```python
from build123d import *

# Parameters (mm, degrees)
SKETCH_1_W          = 18
SKETCH_1_H          = 49
EXTRUDE_1_DEPTH     = 2
CUT_EXTRUDE_1_DEPTH = 0.1


with BuildPart() as part:
    # ｽｹｯﾁ1 → ﾎﾞｽ - 押し出し1 (new body)
    with BuildSketch(Plane.XY):
        with Locations((9, 24.5)):
            Rectangle(SKETCH_1_W, SKETCH_1_H)
    extrude(amount=EXTRUDE_1_DEPTH)

    # ｽｹｯﾁ2 → ｶｯﾄ - 押し出し1 (cut)
    with BuildSketch(Plane.XY.offset(2)):
        with BuildLine():
            Line((15.875, 36.3125), (15.875, 33.870192308))
            Line((15.875, 33.870192308), (7.775315505, 33.870192308))
            Line((7.775315505, 33.870192308), (6.49214994, 27.607008714))
            add(Edge.make_bspline(
                [(6.49214994, 27.607008714), (6.744262228, 27.676611099), (7.232689912, 27.811454712), (7.953595395, 27.961172542), (8.637981636, 28.051424939), (9.082087281, 28.063748319), (9.29698768, 28.069711538)],
                knots=[0, 0, 0, 0, 1.100273476, 2.13160584, 3.095893838, 4, 4, 4, 4], degree=3))
            add(Edge.make_bspline(
                [(9.29698768, 28.069711538), (9.562896695, 28.063956155), (10.085740255, 28.052639632), (10.850726663, 27.943974013), (11.580973668, 27.772932808), (12.27495408, 27.53398783), (12.933951755, 27.228441252), (13.551903557, 26.846761301), (14.138085072, 26.400900602), (14.68198022, 25.888285431), (15.175404531, 25.324122288), (15.609240996, 24.717530344), (15.977740048, 24.074404643), (16.274108756, 23.388600502), (16.510766458, 22.667699833), (16.668282709, 21.904117441), (16.77317139, 21.105050767), (16.784889768, 20.558692889), (16.790865385, 20.280085637)],
                knots=[0, 0, 0, 0, 1.052922333, 2.070308379, 3.05430497, 4.020497103, 4.973039431, 5.925935799, 6.892292201, 7.88610001, 8.88166317, 9.857072816, 10.836096531, 11.812156883, 12.81219415, 13.836441305, 14.89672472, 16, 16, 16, 16], degree=3))
            add(Edge.make_bspline(
                [(16.790865385, 20.280085637), (16.786340497, 20.086032674), (16.777351873, 19.700549205), (16.731641482, 19.128068125), (16.643632414, 18.567706707), (16.525469862, 18.019390612), (16.372100912, 17.48415792), (16.186437884, 16.960476631), (15.959225626, 16.451606182), (15.710001448, 15.952731619), (15.429378088, 15.475131061), (15.117920743, 15.028483492), (14.788862669, 14.606088649), (14.434795386, 14.212476644), (14.052427901, 13.850233968), (13.646390984, 13.517210839), (13.219924628, 13.20777536), (12.766430926, 12.934488174), (12.296015104, 12.683008062), (11.801883841, 12.47669971), (11.295285147, 12.292251296), (10.76892769, 12.145229331), (10.224003714, 12.030027487), (9.659614974, 11.951782329), (9.078721487, 11.894792638), (8.684964705, 11.891225138), (8.486065204, 11.889423077)],
                knots=[0, 0, 0, 0, 1.056347294, 2.098418968, 3.122841568, 4.141288669, 5.149314143, 6.15115421, 7.162517403, 8.180376062, 9.185164535, 10.17417709, 11.141909838, 12.097768115, 13.052685741, 14.0056014, 14.954263652, 15.917497458, 16.885230207, 17.854509472, 18.828990115, 19.81800267, 20.826176721, 21.857883937, 22.917946725, 24, 24, 24, 24], degree=3))
            add(Edge.make_bspline(
                [(8.486065204, 11.889423077), (8.248796225, 11.894123242), (7.781997537, 11.903370263), (7.098098679, 12.000106743), (6.440093951, 12.138654103), (5.813280227, 12.347090153), (5.212040023, 12.608260854), (4.644467603, 12.938344093), (4.096060448, 13.312398352), (3.589112484, 13.753816468), (3.118603926, 14.236296376), (2.697418571, 14.759883184), (2.322313344, 15.315935282), (1.999295101, 15.90715308), (1.72376392, 16.531983085), (1.507308375, 17.192766359), (1.332603853, 17.886050314), (1.258693796, 18.363344733), (1.221153846, 18.605769231)],
                knots=[0, 0, 0, 0, 1.0467383, 2.05933395, 3.04377827, 4.011590433, 4.970194871, 5.932262533, 6.905835911, 7.896367577, 8.894135286, 9.877477877, 10.858688626, 11.851381753, 12.8477658, 13.868841284, 14.917554742, 16, 16, 16, 16], degree=3))
            Line((1.221153846, 18.605769231), (3.358173077, 18.605769231))
            add(Edge.make_bspline(
                [(3.358173077, 18.605769231), (3.410754869, 18.378690153), (3.511819994, 17.942231555), (3.733655534, 17.329016537), (4.004885865, 16.782558961), (4.327404736, 16.295630189), (4.712146908, 15.871026119), (5.151177487, 15.492631465), (5.643400389, 15.151261389), (6.190361469, 14.866717205), (6.767393312, 14.624042293), (7.371327366, 14.46244594), (7.985719437, 14.348820223), (8.401270492, 14.337446279), (8.610088642, 14.331730769)],
                knots=[0, 0, 0, 0, 1.136247022, 2.183929868, 3.172523383, 4.106158343, 5.02341133, 5.958108904, 6.928429099, 7.938127109, 8.96079061, 9.975095812, 10.982467395, 12, 12, 12, 12], degree=3))
            add(Edge.make_bspline(
                [(8.610088642, 14.331730769), (8.813913058, 14.33731499), (9.215245002, 14.348310367), (9.805872472, 14.432940075), (10.376099349, 14.563279979), (10.920299044, 14.758337386), (11.447994518, 14.995405916), (11.945837492, 15.299628129), (12.428230281, 15.64974004), (12.880178833, 16.050855684), (13.294104371, 16.492881642), (13.659837981, 16.96557605), (13.96448091, 17.46983531), (14.221207615, 17.996929439), (14.41615238, 18.552635337), (14.555224056, 19.13434869), (14.636887724, 19.743506323), (14.648121645, 20.158995734), (14.653846154, 20.370718149)],
                knots=[0, 0, 0, 0, 1.027316725, 2.022795036, 3.002884548, 3.971462791, 4.93288096, 5.914575861, 6.907176829, 7.935150275, 8.956128384, 9.956726525, 10.942570165, 11.921478529, 12.907843606, 13.90538589, 14.932640048, 16, 16, 16, 16], degree=3))
            add(Edge.make_bspline(
                [(14.653846154, 20.370718149), (14.649366142, 20.561733531), (14.640597156, 20.935618961), (14.568951668, 21.482620705), (14.444330839, 22.000189082), (14.271357655, 22.490823424), (14.051741719, 22.954986487), (13.783365915, 23.393157308), (13.46119369, 23.799560709), (13.093175662, 24.174386832), (12.690009348, 24.52031357), (12.244758171, 24.815208159), (11.76673974, 25.063293027), (11.261713358, 25.277387801), (10.717666459, 25.431153587), (10.145372942, 25.546595808), (9.53865284, 25.613375329), (9.123834408, 25.622641033), (8.910606971, 25.627403846)],
                knots=[0, 0, 0, 0, 1.045622112, 2.046656509, 3.013763289, 3.955457236, 4.890082067, 5.820317437, 6.762574623, 7.722996705, 8.69280354, 9.665887285, 10.63943826, 11.638615906, 12.663482002, 13.728887084, 14.832589034, 16, 16, 16, 16], degree=3))
            add(Edge.make_bspline(
                [(8.910606971, 25.627403846), (8.726033366, 25.623453753), (8.344935699, 25.615297812), (7.76035361, 25.55524611), (7.146047423, 25.458368054), (6.504372016, 25.32511162), (5.833400345, 25.150728758), (5.134548368, 24.94176046), (4.406346697, 24.691919718), (3.915688608, 24.503241621), (3.663461538, 24.40625)],
                knots=[0, 0, 0, 0, 0.817624296, 1.688186739, 2.600797293, 3.572016777, 4.590301741, 5.671205678, 6.80286297, 8, 8, 8, 8], degree=3))
            Line((3.663461538, 24.40625), (6.105769231, 36.3125))
            Line((6.105769231, 36.3125), (15.875, 36.3125))
        make_face()
    extrude(amount=-CUT_EXTRUDE_1_DEPTH, mode=Mode.SUBTRACT)


solid = part.part
```
The listing builds one solid part. Answer for the finished solid, in the listing's coordinates (mm). Round coordinates to 2 decimals unless told otherwise and drop trailing zeros. Loops run counter-clockwise (first coordinate to the right, second up) from the corner with the lowest first, then second, coordinate; pieces in that order, holes last.
Q1. Find the intervals of material crossed by line 1 (Z direction, x = 9.75, y = 12.5), in increasing order.
Q2. For a pull along X with two mould halves and no side action, classify faces 1 (the face through (18, 24, 1)), 2 (the face through (10, 26, 1.9)), 3 (the face through (0, 24, 1)), 4 (the face through (9, 49, 1)) as released by +X, released by -X, zero draft, split by the parting line, or undercut.
Q3. Section A-A, the plane y = 34.5 is taken. Determine the outline of the cut face in (x, z) (3 decimals).
Completed:
1. line 1: z = 0 to 1.9
2. face 1: released by +X
2. face 2: undercut
2. face 3: released by -X
2. face 4: zero draft
3. outline: (0, 0) - (18, 0) - (18, 2) - (15.875, 2) - (15.875, 1.9) - (5.734, 1.9) - (5.734, 2) - (0, 2) - close
